from build123d import *

# Parameters (mm, degrees)
SKETCH1_W           = 20.32
SKETCH1_H           = 20.32
BOARD_OUTLINE_DEPTH = 1.6
SKETCH2_R           = 0.4
SKETCH2_R_2         = 0.254
NPTH_DEPTH          = 15.45721965
SKETCH3_R           = 0.51
PTH_DEPTH           = 15.45721965


with BuildPart() as part:
    # Sketch1 → Board_Outline (new body)
    with BuildSketch(Plane.XY):
        Rectangle(SKETCH1_W, SKETCH1_H)
    extrude(amount=BOARD_OUTLINE_DEPTH)

    # Sketch2 → NPTH (cut, through all)
    with BuildSketch(Plane.XY):
        with Locations((8.26, -6.448)):
            Circle(SKETCH2_R)
        with Locations((-8.49, -6.448)):
            Circle(SKETCH2_R)
        with Locations((-6.985, 2.413)):
            Circle(SKETCH2_R_2)
        with Locations((-3.04, 0.389)):
            Circle(SKETCH2_R_2)
        with Locations((-6.35, -0.381)):
            Circle(SKETCH2_R_2)
        with Locations((-7.62, -5.08)):
            Circle(SKETCH2_R_2)
        with Locations((-7.62, -0.508)):
            Circle(SKETCH2_R_2)
        with Locations((-8.89, -5.08)):
            Circle(SKETCH2_R_2)
        with Locations((0, -0.508)):
            Circle(SKETCH2_R_2)
        with Locations((2.54, 4.826)):
            Circle(SKETCH2_R_2)
        with Locations((2.54, 0.889)):
            Circle(SKETCH2_R_2)
        with Locations((-1.27, 5.08)):
            Circle(SKETCH2_R_2)
        with Locations((-5.08, -5.461)):
            Circle(SKETCH2_R_2)
        with Locations((8.382, -4.953)):
            Circle(SKETCH2_R_2)
        with Locations((-9.017, -0.381)):
            Circle(SKETCH2_R_2)
        with Locations((9.144, -0.127)):
            Circle(SKETCH2_R_2)
        with Locations((3.81, -0.381)):
            Circle(SKETCH2_R_2)
        with Locations((-6.35, -5.08)):
            Circle(SKETCH2_R_2)
        with Locations((7.62, 1.27)):
            Circle(SKETCH2_R_2)
        with Locations((6.223, 1.27)):
            Circle(SKETCH2_R_2)
        with Locations((6.35, 5.969)):
            Circle(SKETCH2_R_2)
        with Locations((-0.889, -5.08)):
            Circle(SKETCH2_R_2)
    extrude(amount=NPTH_DEPTH, mode=Mode.SUBTRACT)

    # Sketch3 → PTH (cut, through all)
    with BuildSketch(Plane.XY):
        with Locations((8.89, 8.89)):
            Circle(SKETCH3_R)
        with Locations((6.35, 8.89)):
            Circle(SKETCH3_R)
        with Locations((3.81, 8.89)):
            Circle(SKETCH3_R)
        with Locations((1.27, 8.89)):
            Circle(SKETCH3_R)
        with Locations((-1.27, 8.89)):
            Circle(SKETCH3_R)
        with Locations((-3.81, 8.89)):
            Circle(SKETCH3_R)
        with Locations((-6.35, 8.89)):
            Circle(SKETCH3_R)
        with Locations((-8.89, 8.89)):
            Circle(SKETCH3_R)
        with Locations((-8.89, -8.89)):
            Circle(SKETCH3_R)
        with Locations((-6.35, -8.89)):
            Circle(SKETCH3_R)
        with Locations((-3.81, -8.89)):
            Circle(SKETCH3_R)
        with Locations((-1.27, -8.89)):
            Circle(SKETCH3_R)
        with Locations((1.27, -8.89)):
            Circle(SKETCH3_R)
        with Locations((3.81, -8.89)):
            Circle(SKETCH3_R)
        with Locations((6.35, -8.89)):
            Circle(SKETCH3_R)
        with Locations((8.89, -8.89)):
            Circle(SKETCH3_R)
    extrude(amount=PTH_DEPTH, mode=Mode.SUBTRACT)


solid = part.part
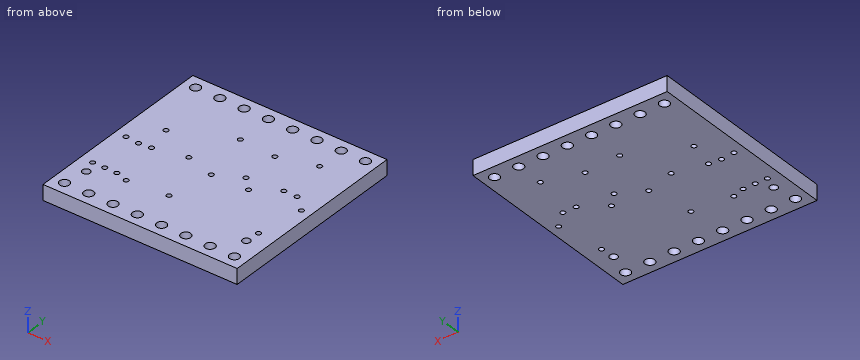
Geometry: final body of the model. Coordinates: model frame, mm. Coordinates: 2 decimals unless noted, no trailing zeros. Write each loop counter-clockwise with the first axis right and the second up, starting at its lowest first coordinate (ties: lowest second). Pieces come first, ordered by that corner, then holes. Notation, with made-up numbers: (34.5, 82.25) - (68.5, 82.25) arc R18 ccw to (68.5, 111.25) - close; hole circle Ø1 at (70.25, 30). An arc over 180 degrees is marked (long way). Return JSON: item names as keys, results as strings.
Item 1: Section query B-B (x = 2.54). Output: boundary loops of the cut face in (y, z) (3 decimals).
Completed:
{"outline": "(-10.16, 0) - (0.635, 0) - (0.635, 1.6) - (-10.16, 1.6) - close; (1.143, 0) - (4.572, 0) - (4.572, 1.6) - (1.143, 1.6) - close; (5.08, 0) - (10.16, 0) - (10.16, 1.6) - (5.08, 1.6) - close"}
Item 2: Section query A-A (x = -3.04). Output: boundary loops of the cut face in (y, z) (3 decimals), and give its area (3 significant figures).
Completed:
{"outline": "(-10.16, 0) - (0.135, 0) - (0.135, 1.6) - (-10.16, 1.6) - close; (0.643, 0) - (10.16, 0) - (10.16, 1.6) - (0.643, 1.6) - close", "area": "31.7 mm2"}
Item 3: Section query C-C (y = 8.89). Count the separate pieces of the cut face and the enclosed holes in it, and give its area (3 significant figures).
Completed:
{"separate pieces": "9", "enclosed holes": "0", "area": "19.5 mm2"}
Item 4: Line query: L1, parallel to Y at x = 3.81, z = 1.15 (3 decimals); L2, parallel to Y at x = -1.27, z = 1.1; L3, parallel to X at y = 1.27, z = 0.95. Output: solid intervals per line, ascending.
Completed:
{"L1": "y = -10.16 to -9.4, -8.38 to -0.635, -0.127 to 8.38, 9.4 to 10.16", "L2": "y = -10.16 to -9.4, -8.38 to 4.83, 5.33 to 8.38, 9.4 to 10.16", "L3": "x = -10.16 to 5.97, 6.48 to 7.37, 7.87 to 10.16"}
Item 5: Section query D-D (x = -6.35). Output: boundary loops of the cut face in (y, z) (3 decimals), and give its area (3 significant figures).
Completed:
{"outline": "(-10.16, 0) - (-9.4, 0) - (-9.4, 1.6) - (-10.16, 1.6) - close; (-8.38, 0) - (-5.334, 0) - (-5.334, 1.6) - (-8.38, 1.6) - close; (-4.826, 0) - (-0.635, 0) - (-0.635, 1.6) - (-4.826, 1.6) - close; (-0.127, 0) - (8.38, 0) - (8.38, 1.6) - (-0.127, 1.6) - close; (9.4, 0) - (10.16, 0) - (10.16, 1.6) - (9.4, 1.6) - close", "area": "27.6 mm2"}
